```python
from build123d import *

# Parameters (mm, degrees)
SKETCH1_R           = 2.5
BOSS_EXTRUDE1_DEPTH = 2.65
SKETCH1_5_W         = 4.5
SKETCH1_5_H         = 2
BOSS_EXTRUDE2_DEPTH = 5
FILLET1_R           = 1
MOVE_FACE1_BY       = 0.1
MOVE_FACE1_2_BY     = 0.1
MOVE_FACE1_3_BY     = 0.1
MOVE_FACE2_BY       = 0.1


with BuildPart() as part:
    # Sketch1 → Boss-Extrude1 (new, symmetric)
    with BuildSketch(Plane(origin=(0, 0, 0), x_dir=(0, 0, -1), z_dir=(1, 0, 0))):
        with BuildLine():
            Line((2.049048496, -11.620731486), (13.669779982, -9.571682989))
            Line((13.669779982, -9.571682989), (29.59, 6.348537029))
            Line((29.59, 6.348537029), (29.59, 63.5))
            ThreePointArc((29.59, 63.5), (25.09, 68), (20.59, 63.5))
            Line((20.59, 63.5), (20.59, 15.59029712))
            Line((20.59, 15.59029712), (9.571682989, 13.669779982))
            Line((9.571682989, 13.669779982), (-2.049048496, 11.620731486))
            ThreePointArc((-2.049048496, 11.620731486), (-11.620731486, -2.049048496), (2.049048496, -11.620731486))
        make_face()
        with Locations((25.09, 63.5)):
            Circle(SKETCH1_R, mode=Mode.SUBTRACT)
        with Locations((25.09, 13.5)):
            Circle(SKETCH1_R, mode=Mode.SUBTRACT)
        with Locations((25.09, 38.5)):
            Circle(SKETCH1_R, mode=Mode.SUBTRACT)
    extrude(amount=BOSS_EXTRUDE1_DEPTH, both=True)

    # Sketch1<5> → Boss-Extrude2 (add)
    with BuildSketch(Plane(origin=(0, 0, 0), x_dir=(0, 0, -1), z_dir=(1, 0, 0))):
        with Locations((22.84, 58)):
            Rectangle(SKETCH1_5_W, SKETCH1_5_H)
    extrude(amount=BOSS_EXTRUDE2_DEPTH)

    # Fillet1
    fillet1_edges = [part.edges().sort_by_distance(p)[0] for p in [
        (2.65, 57, -22.84),
    ]]
    fillet(fillet1_edges, radius=FILLET1_R)

    # Move Face1: a curved face moved outward by 0.1
    add(Solid.thicken(part.faces().sort_by_distance((0, 13.5, -22.59))[0], MOVE_FACE1_BY))

    # Move Face1 2: a curved face moved outward by 0.1
    add(Solid.thicken(part.faces().sort_by_distance((0, 38.5, -22.59))[0], MOVE_FACE1_2_BY))

    # Move Face1 3: a curved face moved outward by 0.1
    add(Solid.thicken(part.faces().sort_by_distance((0, 63.5, -22.59))[0], MOVE_FACE1_3_BY))

    # Move Face2: a face moved inward by 0.1
    extrude(part.faces().sort_by_distance((3.825, 59, -22.84))[0], amount=MOVE_FACE2_BY, dir=(0, -1, 0), mode=Mode.SUBTRACT)


solid = part.part
```
For this review, take the finished solid that the model builds, in its own axes (mm). A direction names the side the tool comes from. Give positions to 0.01 mm unless a question says otherwise; leave off trailing zeros. Order: outer loops, then holes, each group sorted by start corner. A loop starts at its lowest first (then second) coordinate and runs counter-clockwise, first axis right, second up.
1) Take a section at A-A (y = 38.5). Give the boundary of the cut face in (x, z), then the cut area to 3 significant figures.
2) For faces 4 (the face through (4, 58.9, -23)), 5 (the face through (0, 40, -20.59)), 6 (the face through (4, 58, -25.09)), list the 3-axis set-ups (+Z, -Z, +X, -X, +Y, -Y) from which the entire face can be reached by the end or side of a thin tool; tool diameter is ignored.
3) Take a section at C-C (z = -24). Give the boundary of the cut face in (x, y), then the cut area to 3 significant figures.
4) Wall thickness on line 1 (Y direction, x = 0.65, z = -25.09); line 2 (Z direction, x = 1.75, y = 31.5); line 3 (Y direction, x = 1.5, z = -27): over which ranges is each line inside the solid? List them lowest first.
5) Take a section at B-B (x = -1.25). Give the boundary of the cut face in (y, z).
6) Insertion check: pin 1 (1.5 mm diameter, centred on x = -0.5, y = 9, fed in from +Z); pin 2 (1.2 mm diameter, centred on x = 4, z = -22, fed in from +Y); pin 3 (3 mm diameter, centred on x = -1.5, z = -7, fed in from +Y). Each pin has a flat end and moves straight along its axis. Give the tip position at first contact, or say it passes through.
7) Take a section at D-D (z = 0). Give the boundary of the cut face in (x, y).
8) The part is to be moulded in two halves that separate along Z. For faces 1 (the face through (-0.04, 36.37, -26.2)), 2 (the face through (0, 68, -25)), 3 (the face through (5, 58, -23)), say which applies: released by +Z, released by -Z, zero draft, split by the parting line, or undercut.
Derived:
1. outline: (-2.65, -29.59) - (2.65, -29.59) - (2.65, -27.49) - (-2.65, -27.49) - close; (-2.65, -22.69) - (2.65, -22.69) - (2.65, -20.59) - (-2.65, -20.59) - close
1. area: 22.3 mm2
2. face 4: +Z, -Z, +X, +Y
2. face 5: +Z, +X, -X, +Y
2. face 6: -Z, +X, +Y, -Y
3. outline: (-2.65, 0.76) - (2.65, 0.76) - (2.65, 11.36) - (-2.65, 11.36) - close; (-2.65, 15.64) - (2.65, 15.64) - (2.65, 36.36) - (-2.65, 36.36) - close; (-2.65, 40.64) - (2.65, 40.64) - (2.65, 56) arc R1 cw to (3.65, 57) - (5, 57) - (5, 58.9) - (2.65, 58.9) - (2.65, 61.36) - (-2.65, 61.36) - close; (-2.65, 65.64) - (2.65, 65.64) - (2.65, 67.87) - (-2.65, 67.87) - close
3. area: 292 mm2
4. line 1: y = 1.85 to 11.1, 15.9 to 36.1, 40.9 to 61.1, 65.9 to 68
4. line 2: z = -29.59 to -20.59
4. line 3: y = 3.76 to 12.05, 14.95 to 37.05, 39.95 to 62.05, 64.95 to 67.57
5. outline: (-11.62, -2.05) - (-9.57, -13.67) - (6.35, -29.59) - (63.5, -29.59) arc R4.5 ccw to (63.5, -20.59) - (15.59, -20.59) - (13.67, -9.57) - (11.62, 2.05) arc R11.8 ccw to start; hole circle Ø4.8 at (13.5, -25.09); hole circle Ø4.8 at (38.5, -25.09); hole circle Ø4.8 at (63.5, -25.09)
6. pin 1: stops at z = 8.44
6. pin 2: stops at y = 58.9
6. pin 3: stops at y = 13.48
7. outline: (-2.65, -11.8) - (2.65, -11.8) - (2.65, 11.98) - (-2.65, 11.98) - close
8. face 1: undercut
8. face 2: split by the parting line
8. face 3: zero draft
